Design review of the part built by this model. Coordinates are the model's own, in mm. A direction names the side the tool comes from. Give positions to 0.01 mm unless a question says otherwise; leave off trailing zeros. Loops run counter-clockwise (first coordinate to the right, second up) from the corner with the lowest first, then second, coordinate; pieces in that order, holes last. Notation, with made-up numbers: M 60,6.5 L 111,6.5 A4 cw 111,10.5 Z; hole C 68,65.5 d6. An arc over 180 degrees is marked long. Use CSV: the item, a comma, the result in double quotes.
from build123d import *

# Parameters (mm, degrees)
F0_R     = 15
F1_DEPTH = 100
F2_W     = 20
F2_H     = 10
F3_DEPTH = 75


with BuildPart() as f1:
    # F0 (on Top) → F1 (new body)
    with BuildSketch(Plane.XY):
        Circle(F0_R)
    extrude(amount=F1_DEPTH)

    # F2 (on Front) → F3 (cut, symmetric)
    with BuildSketch(Plane.XZ):
        with Locations((0, 72.273272)):
            Rectangle(F2_W, F2_H)
    extrude(amount=F3_DEPTH, both=True, mode=Mode.SUBTRACT)


solid = f1.part
(1) We need section D-D on y = -13. State the section outline as (x, z) points.
A:
outline,"M -7.48,0 L 7.48,0 L 7.48,67.27 L -7.48,67.27 Z; M -7.48,77.27 L 7.48,77.27 L 7.48,100 L -7.48,100 Z"
(2) We need section C-C on z = 45. State the section outline as (x, y) points.
A:
outline,"C 0,0 d30"
(3) Machinability: for faces 1 (the flat face through (10, 0, 72)), 2 (the flat face through (0, 0, 0)), which of the approach directions +Z, -Z, +X, -X, +Y, -Y give a long, thin tool a straight path to every point of the face, cutting with its end or side? Answer none if there is none.
A:
face 1,"+Y, -Y"
face 2,"-Z, +X, -X, +Y, -Y"
(4) The part is to be moulded in two halves that separate along X. For faces 3 (the cylindrical face through (-14.985, 0.66, 49.3)), 4 (the flat face through (-10, 0, 72)), 5 (the flat face through (0, 0, 67.273)), 6 (the flat face through (0, 0, 100)), say which applies: released by +X, released by -X, zero draft, split by the parting line, or undercut.
A:
face 3,"split by the parting line"
face 4,"undercut"
face 5,"undercut"
face 6,"zero draft"
(5) We need section A-A on y = 0. State the section outline as (x, z) points.
A:
outline,"M -15,0 L 15,0 L 15,100 L -15,100 Z; hole M -10,67.27 L 10,67.27 L 10,77.27 L -10,77.27 Z"
(6) We need section B-B on x = 0. State the section outline as (y, z) points, then the cut area to 3 significant figures.
A:
outline,"M -15,0 L 15,0 L 15,67.27 L -15,67.27 Z; M -15,77.27 L 15,77.27 L 15,100 L -15,100 Z"
area,"2,700 mm²"
(7) Wall thickness on line 1 along Z through (x, y) = (3.25, 0); line 2 along X through (y, z) = (-0.5, 87); line 3 along X through (y, z) = (-10, 41): over which ranges is each line inside the solid? List them lowest first. Write a range as [from, to].
A:
line 1,"[0, 67.27], [77.27, 100]"
line 2,"[-14.99, 14.99]"
line 3,"[-11.18, 11.18]"
(8) Clearance check with flat-ended pins moving along their axes: P1, Ø4, axis at x = -11.5, z = 28, coming from the -Y side; P2, Ø8, axis at y = -5, z = 72.5, coming from the -X side; P3, Ø3, axis at y = 2, z = 70, coming from the +X side. State where each tip first meets the part, or that it passes through.
A:
P1,"y = -11.61"
P2,"x = -14.97"
P3,"x = 14.99"
